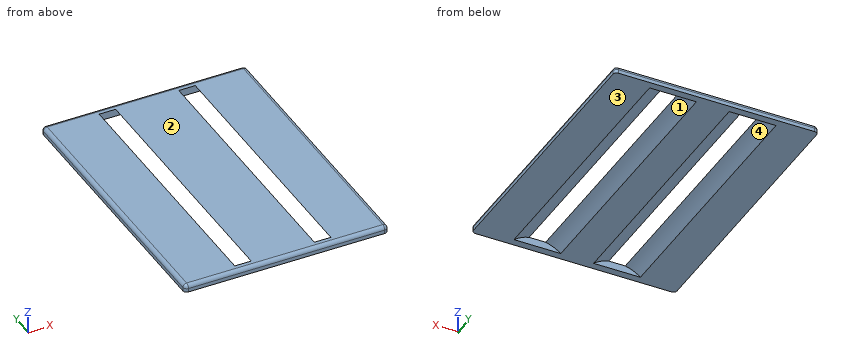
from build123d import *

# Parameters (mm, degrees)
F0_W     = 55
F0_H     = 73
F1_DEPTH = 2
F3_DEPTH = 71
F5_DEPTH = 2
F6_R     = 1


with BuildPart() as f1:
    # F0 (on Top) → F1 (new body)
    with BuildSketch(Plane.XY):
        with Locations((27.5, 36.5)):
            Rectangle(F0_W, F0_H)
    extrude(amount=F1_DEPTH)

    # F2 (on face) → F3 (cut)
    with BuildSketch(Plane.XZ):
        with BuildLine():
            ThreePointArc((36.0279513957, 2), (33.8636583719, 1.2366571717), (31.9303876701, 0))
            Line((31.9303876701, 0), (44.5696123299, 0))
            ThreePointArc((44.5696123299, 0), (42.6363416281, 1.2366571717), (40.4720486043, 2))
            Line((40.4720486043, 2), (36.0279513957, 2))
        make_face()
        with BuildLine():
            Line((10.4303876701, 0), (23.0696123299, 0))
            ThreePointArc((23.0696123299, 0), (21.1363416281, 1.2366571717), (18.9720486043, 2))
            Line((18.9720486043, 2), (14.5279513957, 2))
            ThreePointArc((14.5279513957, 2), (12.3636583719, 1.2366571717), (10.4303876701, 0))
        make_face()
    extrude(amount=-F3_DEPTH, mode=Mode.SUBTRACT)

    # F4 (on face) → F5 (join)
    with BuildSketch(Plane.XY.offset(2)):
        Polygon((55, -2), (55, 0), (40.4720486043, 0), (36.0279513957, 0), (18.9720486043, 0), (14.5279513957, 0), (0, 0), (0, -2), align=None)
    extrude(amount=-F5_DEPTH)

    # F6
    f6_edges = [f1.edges().sort_by_distance(p)[0] for p in [
        (0, 35.5, 2),
        (27.5, 73, 2),
        (55, 35.5, 2),
        (27.5, -2, 2),
        (55, 73, 1),
        (0, 73, 1),
        (0, -2, 1),
        (55, -2, 1),
    ]]
    fillet(f6_edges, radius=F6_R)


solid = f1.part
Could you check a few things on this model? Use its own coordinates, in mm. Face numbers are marked on the shaded views. A direction names the side the tool comes from. Give positions to 0.01 mm unless a question says otherwise; leave off trailing zeros. Write each loop counter-clockwise with the first axis right and the second up, starting at its lowest first coordinate (ties: lowest second). Pieces come first, ordered by that corner, then holes. Notation, with made-up numbers: (56.5, 39.5) - (91.5, 39.5) arc R5 ccw to (91.5, 47.5) - close; hole circle Ø2 at (-40, 26.25). An arc over 180 degrees is marked (long way). Use CSV: the item, a comma, the result in double quotes. Start each with the question number.
Item 1: If I drill on line 1 along Y through (x, z) = (14.5, 0.3); line 2 along X through (y, z) = (18, 1.05); line 3 along X through (y, z) = (42, 0.1), over which ranges is the centre line in solid material (lowest first)?
Item 2: I want a section at B-B, the plane y = 53.5. Please give me the cut outline in (x, z), then the cut area to 3 significant figures.
Item 3: If we mould it in two halves opening along X, with no side actions, what happens to the marked faces 1 and 2? For each: pulls with the +X half, pulls with the -X half, needs draft (parallel to the pull), parting line crosses it, or undercut.
Item 4: I want a section at A-A, the plane x = 38. Please give me the cut outline in (y, z), then the cut area to 3 significant figures.
Item 5: For the marked faces 3 and 4, which set-ups out of +Z, -Z, +X, -X, +Y, -Y let a thin tool reach every point of the face, with its end or its side?
Item 6: I'm going to push flat-ended pins straight in: pin 1 (5 mm diameter, centred on x = 40, y = 17.5, fed in from -Z); pin 2 (1.5 mm diameter, centred on x = 36, y = 55.5, fed in from -Z). Where does each tip first touch, or does it pass through?
Item 7: I want a section at C-C, the plane z = 1.6. Please give me the cut outline in (x, y), then the cut area to 3 significant figures.
Item 8: I want a section at D-D, the plane x = 43.5. Please give me the cut outline in (y, z).
Findings:
1,line 1,"y = -2 to 0, 71 to 73"
1,line 2,"x = 0 to 12, 21.5 to 33.5, 43 to 55"
1,line 3,"x = 0 to 10.56, 22.94 to 32.06, 44.44 to 55"
2,outline,"(0, 0) - (10.43, 0) arc R10 cw to (14.53, 2) - (1, 2) arc R1 ccw to (0, 1) - close; (18.97, 2) arc R10 cw to (23.07, 0) - (31.93, 0) arc R10 cw to (36.03, 2) - close; (40.47, 2) arc R10 cw to (44.57, 0) - (55, 0) - (55, 1) arc R1 ccw to (54, 2) - close"
2,area,"72.2 mm2"
3,face 1,"undercut"
3,face 2,"needs draft"
4,outline,"(-2, 0) - (0, 0) - (0, 2) - (-1, 2) arc R1 ccw to (-2, 1) - close; (71, 0) - (73, 0) - (73, 1) arc R1 ccw to (72, 2) - (71, 2) - close"
4,area,"7.57 mm2"
5,face 3,"-Z, +X, -X, +Y, -Y"
5,face 4,"-Z"
6,pin 1,"stops at z = 1.3"
6,pin 2,"stops at z = 1.79"
7,outline,"(0.2, -1) arc R0.8 ccw to (1, -1.8) - (54, -1.8) arc R0.8 ccw to (54.8, -1) - (54.8, 72) arc R0.8 ccw to (54, 72.8) - (1, 72.8) arc R0.8 ccw to (0.2, 72) - close; hole (13.2, 0) - (20.3, 0) - (20.3, 71) - (13.2, 71) - close; hole (34.7, 0) - (41.8, 0) - (41.8, 71) - (34.7, 71) - close"
7,area,"3,070 mm2"
8,outline,"(-2, 0) - (0, 0) - (0, 0.76) - (71, 0.76) - (71, 0) - (73, 0) - (73, 1) arc R1 ccw to (72, 2) - (-1, 2) arc R1 ccw to (-2, 1) - close"
